Read the model definition and answer for the solid it produces. Units are mm, in the model's axes. A direction names the side the tool comes from. Round coordinates to 2 decimals unless told otherwise and drop trailing zeros. Order: outer loops, then holes, each group sorted by start corner. A loop starts at its lowest first (then second) coordinate and runs counter-clockwise, first axis right, second up. Notation, with made-up numbers: (50, 49) - (100, 49) arc R19 cw to (100, 73) - close; hole circle Ø1 at (47.5, -7.75). An arc over 180 degrees is marked (long way). Answer as a JSON object with one key per item and string values. Group by question number.
Q1. Consider line 1 (X direction, y = -11, z = -6.5); line 2 (Y direction, x = -5, z = -1); line 3 (Y direction, x = -15, z = 0). Determine where each line is inside the solid, lowest interval first.
Q2. A cutting plane is placed at D-D on x = 1.5. Determine the outline of the cut face in (y, z).
Q3. A cutting plane is placed at A-A on y = -15. Determine the outline of the cut face in (x, z), and give its area (3 significant figures).
Q4. A tool of negligible diameter and unlimited length cuts with its end or side. For faces 4 (the flat face through (-7, -11.775, 0)), 5 (the flat face through (6, 0, -10.1)), 6 (the flat face through (7, 16, 2.4)), 7 (the flat face through (-12.87, -0.28, -25.95)), from which of +Z, -Z, +X, -X, +Y, -Y can it reach the whole face along a straight path? Write none if from no direction.
Q5. Given pin 1 Ø1 at (y, z) = (1.5, 1.5) entering from -X; pin 2 Ø4 at (x, y) = (-9.5, -7) entering from -Z; pin 3 Ø5 at (x, y) = (-6, -14.5) entering from -Z, each flat-ended and moving along its own axis, determine where each tip first touches the part or whether it passes through.
Q6. A cutting plane is placed at C-C on z = -21.5. Determine the outline of the cut face in (x, y), and give its area (3 significant figures).
Q7. A cutting plane is placed at B-B on z = 0. Count the separate pieces of the cut face and the enclosed holes in it, and give its area (3 significant figures).
Q8. The mould has two halves that part along X. Classify faces 1 (the cylindrical face through (-14.878, -0.28, -23.827)), 2 (the cylindrical face through (-12.22, 2.23, -0.29)), 3 (the flat face through (10.1, 0, -4)): pulls with the +X half, pulls with the -X half, needs draft (parallel to the pull), parting line crosses it, or undercut.
```python
from build123d import *

# Parameters (mm, degrees)
BOSS_EXTRU_1_DEPTH                                = 20
CHAMBRAGE_POUR_VIS_SIX_PANS_CREUX_M41_D           = 4.5
CHAMBRAGE_POUR_VIS_SIX_PANS_CREUX_M41_DEPTH       = 11.55
CHAMBRAGE_POUR_VIS_SIX_PANS_CREUX_M41_CBORE_D     = 8
CHAMBRAGE_POUR_VIS_SIX_PANS_CREUX_M41_CBORE_DEPTH = 1
ESQUISSE6_W                                       = 20.2
ESQUISSE6_H                                       = 23.55054775
ENL_V_MAT_EXTRU_1_DEPTH                           = 3
BOSS_EXTRU_3_DEPTH                                = 40
CONG_1_R                                          = 10


with BuildPart() as part:
    # Base → Boss.-Extru.1 (new, symmetric)
    with BuildSketch(Plane(origin=(0, 0, 0), x_dir=(1, 0, 0), z_dir=(0, 1, 0))):
        Polygon((-3.85, -2.4), (-3.85, 2.4), (-10.1, 2.4), (-10.1, 10.1), (-2.4, 10.1), (-2.4, 3.85), (2.4, 3.85), (2.4, 10.1), (10.1, 10.1), (10.1, 2.4), (3.85, 2.4), (3.85, -2.4), (10.1, -2.4), (10.1, -6.25), (15.4, -6.25), (15.4, 15.4), (-15.4, 15.4), (-15.4, -6.25), (-10.1, -6.25), (-10.1, -2.4), align=None)
    extrude(amount=BOSS_EXTRU_1_DEPTH, both=True)

    # Chambrage pour vis à six pans creux M41
    with Locations(Plane(origin=(15.4, 0, 0), x_dir=(0, 0, -1), z_dir=(1, 0, 0))):
        with Locations((0, 0)):
            chambrage_pour_vis_six_pans_creux_m41 = CounterBoreHole(CHAMBRAGE_POUR_VIS_SIX_PANS_CREUX_M41_D / 2, CHAMBRAGE_POUR_VIS_SIX_PANS_CREUX_M41_CBORE_D / 2, CHAMBRAGE_POUR_VIS_SIX_PANS_CREUX_M41_CBORE_DEPTH, depth=CHAMBRAGE_POUR_VIS_SIX_PANS_CREUX_M41_DEPTH)

    # Symétrie1: Chambrage pour vis à six pans creux M41 across plane
    add(chambrage_pour_vis_six_pans_creux_m41.mirror(Plane(origin=(0, 0, 0), x_dir=(0, 0, 1), z_dir=(1, 0, 0))), mode=Mode.SUBTRACT)

    # Esquisse6 → Enlèv. mat.-Extru.1 (cut, symmetric)
    with BuildSketch(Plane.XY):
        Rectangle(ESQUISSE6_W, ESQUISSE6_H)
    extrude(amount=ENL_V_MAT_EXTRU_1_DEPTH, both=True, mode=Mode.SUBTRACT)

    # Esquisse14 → Boss.-Extru.3 (add)
    with BuildSketch(Plane.XZ.offset(20)):
        with BuildLine():
            Line((-15.4, -15.4), (15.4, -15.4))
            Line((15.4, -15.4), (15.4, -17.9))
            Line((15.4, -17.9), (15.4, -20.835156926))
            ThreePointArc((15.4, -20.835156926), (14.892113101, -23.787279745), (13.42685396, -26.399940055))
            Line((13.42685396, -26.399940055), (12.329607692, -25.509925555))
            ThreePointArc((12.329607692, -25.509925555), (12.644690295, -23.181973462), (12.75, -20.835156926))
            Line((12.75, -20.835156926), (12.75, -17.87758102))
            Line((12.75, -17.87758102), (-12.75, -17.87758102))
            Line((-12.75, -17.87758102), (-12.75, -20.835156926))
            ThreePointArc((-12.75, -20.835156926), (-12.644690295, -23.181973462), (-12.329607692, -25.509925555))
            Line((-12.329607692, -25.509925555), (-13.42685396, -26.399940055))
            ThreePointArc((-13.42685396, -26.399940055), (-14.892113101, -23.787279745), (-15.4, -20.835156926))
            Line((-15.4, -20.835156926), (-15.4, -17.9))
            Line((-15.4, -17.9), (-15.4, -15.4))
        make_face()
    extrude(amount=-BOSS_EXTRU_3_DEPTH)

    # Congé1
    # the kernel refuses this fillet: 10 mm, written as the material it adds along each edge
    with BuildSketch(Plane(origin=(-12.75, -20, -17.87758102), x_dir=(0, 0, -1), z_dir=(0, 1, 0))) as cong_1_piece_1:
        with BuildLine():
            CenterArc((10, -7.099595966), CONG_1_R, 134.768371909, 45.231628091)
            Line((0, -7.099595966), (0, 0))
            Line((0, 0), (2.957575906, 0))
        make_face()
    extrude(amount=40)
    with BuildSketch(Plane(origin=(12.75, -20, -17.87758102), x_dir=(-1, 0, 0), z_dir=(0, 1, 0))) as cong_1_piece_2:
        with BuildLine():
            CenterArc((7.099595966, -10), CONG_1_R, 90, 45.231628091)
            Line((0, -2.957575906), (0, 0))
            Line((0, 0), (7.099595966, 0))
        make_face()
    extrude(amount=40)


solid = part.part
```
Result set:
{
 "1": {"line 1": "x = -15.4 to -10.1, -2.4 to 2.4, 10.1 to 15.4", "line 2": "y = -20 to -11.78, 11.78 to 20", "line 3": "y = -20 to -4, 4 to 20"},
 "2": {"outline": "(-20, -17.88) - (20, -17.88) - (20, -3.85) - (-20, -3.85) - close"},
 "3": {"outline": "(-15.4, -20.84) arc R8.83 ccw to (-13.43, -26.4) - (-12.33, -25.51) arc R26.2 cw to (-12.75, -20.84) arc R10 cw to (-5.65, -17.88) - (5.65, -17.88) arc R10 cw to (12.75, -20.84) arc R26.2 cw to (12.33, -25.51) - (13.43, -26.4) arc R8.83 ccw to (15.4, -20.84) - (15.4, 6.25) - (10.1, 6.25) - (10.1, 2.4) - (3.85, 2.4) - (3.85, -2.4) - (10.1, -2.4) - (10.1, -10.1) - (2.4, -10.1) - (2.4, -3.85) - (-2.4, -3.85) - (-2.4, -10.1) - (-10.1, -10.1) - (-10.1, -2.4) - (-3.85, -2.4) - (-3.85, 2.4) - (-10.1, 2.4) - (-10.1, 6.25) - (-15.4, 6.25) - close", "area": "555 mm²"},
 "4": {"face 4": "+Z", "face 5": "+Y, -Y", "face 6": "+Z, +Y, -Y", "face 7": "-Z, +Y, -Y"},
 "5": {"pin 1": "stops at x = -14.4", "pin 2": "stops at z = -19.77", "pin 3": "stops at z = -18.29"},
 "6": {"outline": "(-15.37, -20) - (-12.74, -20) - (-12.74, 20) - (-15.37, 20) - close; (12.74, -20) - (15.37, -20) - (15.37, 20) - (12.74, 20) - close", "area": "211 mm²"},
 "7": {"separate pieces": "4", "enclosed holes": "0", "area": "575 mm²"},
 "8": {"face 1": "pulls with the -X half", "face 2": "needs draft", "face 3": "undercut"}
}
